Source: three-view drawing plus pictorial views. Frame: mm from the lowest corner of the part. Give positions to 0.01 mm unless a question says otherwise; leave off trailing zeros. Write each loop counter-clockwise with the first axis right and the second up, starting at its lowest first coordinate (ties: lowest second). Pieces come first, ordered by that corner, then holes. Notation, with made-up numbers: (30.25, 76) - (37.25, 76) arc R17 cw to (37.25, 99) - close; hole circle Ø5 at (-6.5, -40). An arc over 180 degrees is marked (long way). One line per question, with ' | ' between items. Start each with the question number.
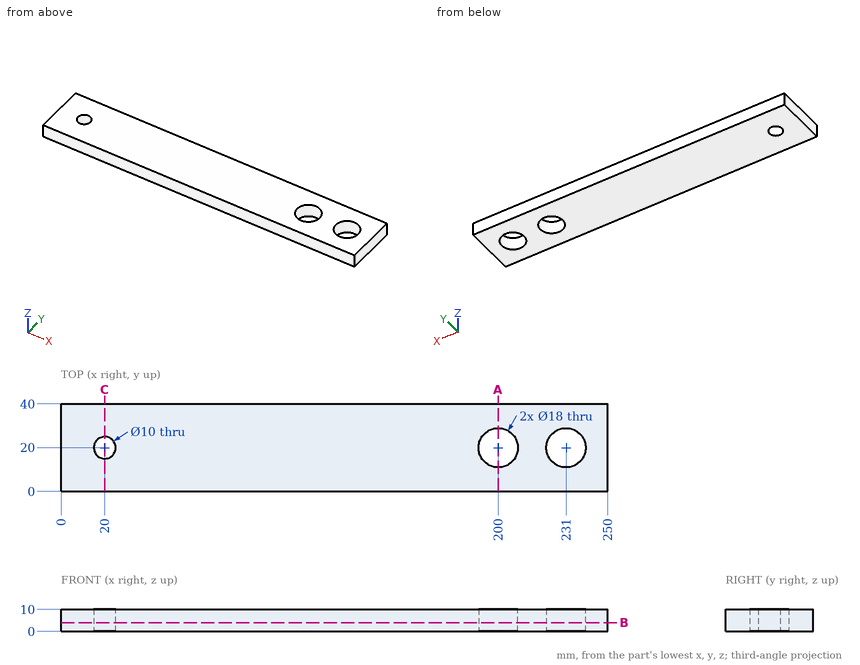
1) Section B-B, the plane z = 4. Output: boundary loops of the cut face in (x, y).
2) Line query: L1, parallel to Y at x = 231, z = 6; L2, parallel to X at y = 13.5, z = 8.75; L3, parallel to Y at x = 21.5, z = 8.25. Output: solid intervals per line, ascending.
3) Section C-C, the plane x = 20. Output: boundary loops of the cut face in (y, z), plus the area to 3 significant figures.
4) Section A-A, the plane x = 200. Output: boundary loops of the cut face in (y, z), plus the area to 3 significant figures.
Answer key:
1) outline: (0, 0) - (250, 0) - (250, 40) - (0, 40) - close; hole circle Ø10 at (20, 20); hole circle Ø18 at (200, 20); hole circle Ø18 at (231, 20)
2) L1: 0 to 11, 29 to 40 | L2: 0 to 193.78, 206.22 to 224.78, 237.22 to 250 | L3: 0 to 15.23, 24.77 to 40
3) outline: (0, 0) - (15, 0) - (15, 10) - (0, 10) - close; (25, 0) - (40, 0) - (40, 10) - (25, 10) - close | area: 300 mm^2
4) outline: (0, 0) - (11, 0) - (11, 10) - (0, 10) - close; (29, 0) - (40, 0) - (40, 10) - (29, 10) - close | area: 220 mm^2
